```python
from build123d import *

# Parameters (mm, degrees)
SKETCH_1_W                = 95.5
SKETCH_1_H                = 121
EXTRUDE_1_DEPTH           = 24.125
CUT_EXTRUDE_START         = -3.125
SKETCH_2_W                = 40
SKETCH_2_H                = 70
SKETCH_2_H_2              = 99.5
CUT_EXTRUDE_1_DEPTH       = 3.125
CUT_EXTRUDE_2_DEPTH       = 3.125
HOLE_WIZARD_M3_1_D        = 2.5
HOLE_WIZARD_M3_1_DEPTH    = 5
HOLE_WIZARD_M3_1_TIP      = 0.751075774
HOLE_WIZARD_M4_1_D        = 3.3
HOLE_WIZARD_M4_1_DEPTH    = 5
HOLE_WIZARD_M4_1_TIP      = 0.991420021
MM_2_D                    = 2
MM_2_DEPTH                = 5
MM_2_TIP                  = 0.600860619
CUT_EXTRUDE_12_DEPTH      = 5
SKETCH_27_W               = 49
SKETCH_27_H               = 45
CUT_EXTRUDE_15_DEPTH      = 25.125
CUT_EXTRUDE_16_DEPTH      = 16
CUT_EXTRUDE_17_DEPTH      = 16
FILLET_2_R                = 5
SKETCH_42_W               = 5
SKETCH_42_H               = 5
CUT_EXTRUDE_24_DEPTH      = 3.125
HOLE_WIZARD_2_D           = 6.6
HOLE_WIZARD_2_CBORE_D     = 11
HOLE_WIZARD_2_CBORE_DEPTH = 8
SKETCH_49_W               = 3
SKETCH_49_H               = 11
CUT_EXTRUDE_28_DEPTH      = 96.5
SKETCH_50_W               = 3
SKETCH_50_H               = 3
CUT_EXTRUDE_29_DEPTH      = 4
CUT_EXTRUDE_29_DEPTH_BACK = 13
SKETCH_52_W               = 3
SKETCH_52_H               = 15
CUT_EXTRUDE_30_DEPTH      = 96.5
PATTERN_LINEAR_4_COUNT    = 16
PATTERN_LINEAR_4_PITCH    = 5.733333333
MM_3_D                    = 4
MM_3_DEPTH                = 5
MM_3_TIP                  = 1.201721238


with BuildPart() as part:
    # 草图1 → 凸台-拉伸1 (new body)
    with BuildSketch(Plane(origin=(0, 0, 0), x_dir=(1, 0, 0), z_dir=(0, 1, 0))):
        with Locations((-170.498130707, -443.224508868)):
            Rectangle(SKETCH_1_W, SKETCH_1_H)
    extrude(amount=EXTRUDE_1_DEPTH)

    # 草图2 → 切除-拉伸1 (cut)
    with BuildSketch(Plane(origin=(0, 24.125, 0), x_dir=(1, 0, 0), z_dir=(0, 1, 0)).offset(CUT_EXTRUDE_START)):
        with Locations((-195.248130707, -465.724508868)):
            Rectangle(SKETCH_2_W, SKETCH_2_H)
        with Locations((-145.248130707, -435.474508868)):
            Rectangle(SKETCH_2_W, SKETCH_2_H_2)
    extrude(amount=CUT_EXTRUDE_1_DEPTH, mode=Mode.SUBTRACT)

    # 草图4 → 切除-拉伸2 (cut)
    with BuildSketch(Plane(origin=(0, 24.125, 0), x_dir=(1, 0, 0), z_dir=(0, 1, 0))):
        Polygon((-165.248130707, -385.724508868), (-166.248130707, -385.724508868), (-166.248130707, -430.724508868), (-175.248130707, -430.724508868), (-175.248130707, -500.724508868), (-215.248130707, -500.724508868), (-218.248130707, -500.724508868), (-218.248130707, -503.724508868), (-122.748130707, -503.724508868), (-122.748130707, -485.224508868), (-125.248130707, -485.224508868), (-165.248130707, -485.224508868), align=None)
    extrude(amount=-CUT_EXTRUDE_2_DEPTH, mode=Mode.SUBTRACT)

    # M3 螺纹孔1
    with Locations(Plane(origin=(-210.248130707, 21, 433.724508868), x_dir=(0, 0, 1), z_dir=(0, 1, 0))):
        with Locations((0, 0), (0, 30), (64, 30), (64, 0)):
            Hole(HOLE_WIZARD_M3_1_D / 2, depth=HOLE_WIZARD_M3_1_DEPTH)
            with Locations((0, 0, -(HOLE_WIZARD_M3_1_DEPTH + HOLE_WIZARD_M3_1_TIP / 2))):  # 118° drill point
                Cone(0, HOLE_WIZARD_M3_1_D / 2, HOLE_WIZARD_M3_1_TIP, mode=Mode.SUBTRACT)

    # M4 螺纹孔1
    with Locations(Plane(origin=(-160.248130707, 21, 390.724508868), x_dir=(0, 0, 1), z_dir=(0, 1, 0))):
        with Locations((0, 0), (0, 30), (90, 0), (90, 30)):
            Hole(HOLE_WIZARD_M4_1_D / 2, depth=HOLE_WIZARD_M4_1_DEPTH)
            with Locations((0, 0, -(HOLE_WIZARD_M4_1_DEPTH + HOLE_WIZARD_M4_1_TIP / 2))):  # 118° drill point
                Cone(0, HOLE_WIZARD_M4_1_D / 2, HOLE_WIZARD_M4_1_TIP, mode=Mode.SUBTRACT)

    # 大小mm 暗销孔2
    with Locations(Plane(origin=(-136.748130707, 21, 480.724508868), x_dir=(0, 0, 1), z_dir=(0, 1, 0))):
        with Locations((0, 0)):
            Hole(MM_2_D / 2, depth=MM_2_DEPTH)
            with Locations((0, 0, -(MM_2_DEPTH + MM_2_TIP / 2))):  # 118° drill point
                Cone(0, MM_2_D / 2, MM_2_TIP, mode=Mode.SUBTRACT)

    # 草图24 → 切除-拉伸12 (cut)
    with BuildSketch(Plane(origin=(0, 21, 0), x_dir=(1, 0, 0), z_dir=(0, 1, 0))):
        with BuildLine():
            Line((-134.248130707, -405.724508868), (-134.248130707, -404.724508868))
            ThreePointArc((-134.248130707, -404.724508868), (-133.248130707, -403.724508868), (-132.248130707, -404.724508868))
            Line((-132.248130707, -404.724508868), (-132.248130707, -405.724508868))
            ThreePointArc((-132.248130707, -405.724508868), (-133.248130707, -406.724508868), (-134.248130707, -405.724508868))
        make_face()
    extrude(amount=-CUT_EXTRUDE_12_DEPTH, mode=Mode.SUBTRACT)

    # 草图27 → 切除-拉伸15 (cut, through all)
    with BuildSketch(Plane(origin=(0, 24.125, 0), x_dir=(1, 0, 0), z_dir=(0, 1, 0))):
        with Locations((-193.748130707, -405.224508868)):
            Rectangle(SKETCH_27_W, SKETCH_27_H)
    extrude(amount=-CUT_EXTRUDE_15_DEPTH, mode=Mode.SUBTRACT)

    # 草图28 → 切除-拉伸16 (cut)
    with BuildSketch(Plane(origin=(0, 0, 0), x_dir=(1, 0, 0), z_dir=(0, 1, 0))):
        Polygon((-151.605995083, -389.724508869), (-171.714464048, -409.832977834), (-185.669197391, -395.878244492), (-165.560728425, -375.769775526), align=None)
    extrude(amount=CUT_EXTRUDE_16_DEPTH, mode=Mode.SUBTRACT)

    # 草图29 → 切除-拉伸17 (cut)
    with BuildSketch(Plane.XZ):
        Polygon((-151.605995083, 389.724508869), (-158.605995083, 382.724508868), (-155.777567958, 382.724508868), (-148.777567958, 389.724508869), (-167.833917144, 408.780858055), (-169.248130707, 410.195071617), (-169.248130707, 407.366644492), align=None)
    extrude(amount=-CUT_EXTRUDE_17_DEPTH, mode=Mode.SUBTRACT)

    # 圆角2
    fillet_2_edges = [part.edges().sort_by_distance(p)[0] for p in [
        (-148.777567958, 8, 389.724508869),
    ]]
    fillet(fillet_2_edges, radius=FILLET_2_R)

    # 草图42 → 切除-拉伸24 (cut)
    with BuildSketch(Plane(origin=(0, 24.125, 0), x_dir=(1, 0, 0), z_dir=(0, 1, 0))):
        with Locations((-166.748130707, -385.224508868)):
            Rectangle(SKETCH_42_W, SKETCH_42_H)
        with Locations((-125.248130707, -385.224508868)):
            Rectangle(SKETCH_42_W, SKETCH_42_H)
        with Locations((-215.748130707, -430.224508868)):
            Rectangle(SKETCH_42_W, SKETCH_42_H)
    extrude(amount=-CUT_EXTRUDE_24_DEPTH, mode=Mode.SUBTRACT)

    # 打孔尺寸(%根据)内六角圆柱头螺钉的类型2 (through all)
    with Locations(Plane(origin=(-165.748130707, 21, 494.724508868), x_dir=(0, 0, 1), z_dir=(0, 1, 0))):
        with Locations((0, 0), (-103, 22.5)):
            CounterBoreHole(HOLE_WIZARD_2_D / 2, HOLE_WIZARD_2_CBORE_D / 2, HOLE_WIZARD_2_CBORE_DEPTH)

    # 草图49 → 切除-拉伸28 (cut, through all)
    with BuildSketch(Plane(origin=(-122.748130707, 0, 0), x_dir=(0, 0, -1), z_dir=(1, 0, 0))):
        with Locations((-502.224508868, 8.5)):
            Rectangle(SKETCH_49_W, SKETCH_49_H)
        with Locations((-384.224508868, 8.5)):
            Rectangle(SKETCH_49_W, SKETCH_49_H)
    extrude(amount=-CUT_EXTRUDE_28_DEPTH, mode=Mode.SUBTRACT)

    # 草图50 → 切除-拉伸29 (cut, two sides)
    with BuildSketch(Plane.XZ.offset(-3)) as cut_extrude_29_sk:
        with Locations((-154.277567958, 384.224508868)):
            Rectangle(SKETCH_50_W, SKETCH_50_H)
    extrude(amount=CUT_EXTRUDE_29_DEPTH, mode=Mode.SUBTRACT)
    extrude(cut_extrude_29_sk.sketch, amount=-CUT_EXTRUDE_29_DEPTH_BACK, mode=Mode.SUBTRACT)

    # 草图52 → 切除-拉伸30 (cut, through all)
    with BuildSketch(Plane(origin=(-122.748130707, 0, 0), x_dir=(0, 0, -1), z_dir=(1, 0, 0))):
        with Locations((-400.224508868, 7.5)):
            Rectangle(SKETCH_52_W, SKETCH_52_H)
    cut_extrude_30 = extrude(amount=-CUT_EXTRUDE_30_DEPTH, mode=Mode.SUBTRACT)

    # 阵列(线性)4: 切除-拉伸30 ×16
    with Locations(*[(0, 0, i * PATTERN_LINEAR_4_PITCH) for i in range(1, PATTERN_LINEAR_4_COUNT)]):
        add(cut_extrude_30, mode=Mode.SUBTRACT)

    # 大小mm 暗销孔3
    with Locations(Plane(origin=(-155.748130707, 0, 494.724508868), x_dir=(0, 0, -1), z_dir=(0, -1, 0))):
        with Locations((0, 0), (103, 22.5)):
            Hole(MM_3_D / 2, depth=MM_3_DEPTH)
            with Locations((0, 0, -(MM_3_DEPTH + MM_3_TIP / 2))):  # 118° drill point
                Cone(0, MM_3_D / 2, MM_3_TIP, mode=Mode.SUBTRACT)


solid = part.part
```
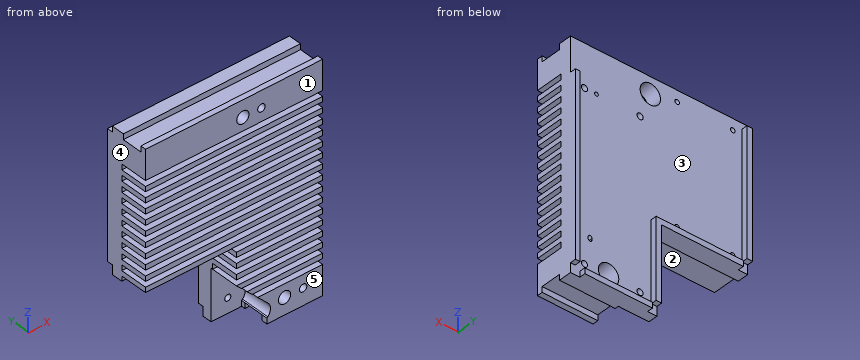
Design review of the part built by this model. Coordinates are the model's own, in mm. Face numbers are marked on the shaded views. A direction names the side the tool comes from. Coordinates: 2 decimals unless noted, no trailing zeros. Order: outer loops, then holes, each group sorted by start corner. A loop starts at its lowest first (then second) coordinate and runs counter-clockwise, first axis right, second up. Notation, with made-up numbers: (7, -32.75) -> (26, -32.75) arc R21 cw to (26, -19.75) -> close; hole circle Ø7 at (21.5, 16). An arc over 180 degrees is marked (long way). One line per item, written item: value. Start each with the question number.
Q1. Tool access review of the marked faces 1 and 2: name each direction out of +Z, -Z, +X, -X, +Y, -Y from which nothing blocks a thin tool from reaching the whole face with its end or side.
Q2. Mouldability with a two-part tool opening along X and no side actions: class the marked faces 3, 4 and 5 as pulls with the +X half, pulls with the -X half, needs draft (parallel to the pull), parting line crosses it, or undercut.
Q3. Take a section at A-A, the plane z = 437.5. State the section outline as (x, y) points (3 decimals), then the cut area to 3 significant figures.
Q4. For probe 1 along Z at (x, y) = (-170.5, 22.5); probe 2 along Y at (x, z) = (-204, 475); probe 3 along Z at (x, y) = (-176, 16.75), list the stretches that pass through material, from the lowest coordinate up.
Q5. Insertion check: pin 1 Ø4.5 at (x, z) = (-160.25, 390.72) entering from +Y; pin 2 Ø2.5 at (y, z) = (22.5, 429) entering from -X; pin 3 Ø4 at (x, y) = (-202, 8) entering from -Z. Each pin has a flat end and moves straight along its axis. Give the tip position at first contact, or say it passes through.
Q6. Take a section at B-B, the plane y = 10. Give the number of separate pieces and of enclosed holes in the cut face, then the cut area to 3 significant figures.
Values follow:
1. face 1: +Z, -Z, +X, -X, -Y
1. face 2: +X, -X, -Y
2. face 3: undercut
2. face 4: pulls with the -X half
2. face 5: needs draft
3. outline: (-218.248, 0) -> (-122.748, 0) -> (-122.748, 24.125) -> (-125.248, 24.125) -> (-125.248, 21) -> (-215.248, 21) -> (-215.248, 24.125) -> (-218.248, 24.125) -> close
3. area: 2,020 mm2
4. probe 1: z = 427.72 to 430.72
4. probe 2: y = 15 to 21
4. probe 3: z = 427.72 to 503.72
5. pin 1: stops at y = 21
5. pin 2: stops at x = -213.25
5. pin 3: stops at z = 430.39
6. separate pieces: 17
6. enclosed holes: 2
6. area: 4,790 mm2
